Read the model definition and answer for the solid it produces. Units are mm, in the model's axes. A direction names the side the tool comes from. Coordinates: 2 decimals unless noted, no trailing zeros. Order: outer loops, then holes, each group sorted by start corner. A loop starts at its lowest first (then second) coordinate and runs counter-clockwise, first axis right, second up.
Autodesk Inventor part; units mm, degrees
ref_plane "YZ Plane" through (0, 0, 0) normal (1, 0, 0) x (0, 1, 0)
ref_plane "XZ Plane" through (0, 0, 0) normal (0, 1, 0) x (-1, 0, 0)
ref_plane "XY Plane" through (0, 0, 0) normal (0, 0, 1) x (1, 0, 0)
ref_plane "Work Plane1" through (0, 0, 0) normal (0, 0, 1) x (1, 0, 0)
sketch "Sketch1" plane through (0, 0, 0) normal (0, 0, 1) x (1, 0, 0)
  circle A0 centre (0, 24.15) radius 1.6 construction
  circle A1 centre (0, -24.15) radius 1.6 construction
  line L0 (-19.85, -7.6776) -> (-19.85, 7.6776) construction
  arc A2 (-19.85, -7.6776) -> (-19.2715, -9.0845) centre (-17.85, -7.6776) ccw construction
  line L1 (-2.2034, -26.3306) -> (-19.2715, -9.0845) construction
  arc A3 (-2.2034, -26.3306) -> (2.2034, -26.3306) centre (0, -24.15) ccw construction
  line L2 (19.2715, -9.0845) -> (2.2034, -26.3306) construction
  arc A4 (19.2715, -9.0845) -> (19.85, -7.6776) centre (17.85, -7.6776) ccw construction
  line L3 (19.85, 7.6776) -> (19.85, -7.6776) construction
  arc A5 (19.85, 7.6776) -> (19.2715, 9.0845) centre (17.85, 7.6776) ccw construction
  line L4 (2.2034, 26.3306) -> (19.2715, 9.0845) construction
  arc A6 (2.2034, 26.3306) -> (-2.2034, 26.3306) centre (0, 24.15) ccw construction
  line L5 (-19.2715, 9.0845) -> (-2.2034, 26.3306) construction
  arc A7 (-19.2715, 9.0845) -> (-19.85, 7.6776) centre (-17.85, 7.6776) ccw construction
  circle A8 centre (0, 0) radius 13.8 construction
  circle A9 centre (0, 0) radius 14.3 construction
  line L6 (-19.85, -27.25) -> (19.85, -27.25)
  line L7 (19.85, -27.25) -> (19.85, 27.25)
  line L8 (19.85, 27.25) -> (-19.85, 27.25)
  line L9 (-19.85, 27.25) -> (-19.85, -27.25)
  circle A10 centre (0, -24.15) radius 1.5
  circle A11 centre (0, 24.15) radius 1.5
  line L10 (14.85, 22.25) -> (14.85, -22.25)
  line L11 (14.85, -22.25) -> (-14.85, -22.25)
  line L12 (-14.85, -22.25) -> (-14.85, 22.25)
  line L13 (-14.85, 22.25) -> (14.85, 22.25)
  dimension "d0" = 0.5
  dimension "d2" = 3
  dimension "d3" = 3
  dimension "d4" = 5
extrude "Extrusion1" add sketch "Sketch1" along normal blind 50
sketch "Sketch2" plane through (-19.85, -27.25, 0) normal (-1, 0, 0) x (0, 0, 1)
  line L0 (50, 54.5) -> (50, 0)
  line L1 (50, 0) -> (50, 54.5)
  circle A0 centre (50, 27.25) radius 15
  point P0 (0, 27.25)
  point P1 (50, 12.25)
  point P2 (50, 42.25)
  dimension "d7" = 30
extrude "Extrusion2" cut sketch "Sketch2" against normal up to surface (34.7 mm away) contours L0 A0 picked at (45.0365, 27.8527)
sketch "Sketch3" plane through (0, 0, 50) normal (0, 0, 1) x (1, 0, 0)
  line L0 (19.85, 27.25) -> (-19.85, 27.25)
  line L1 (-19.85, 27.25) -> (19.85, 27.25)
  line L2 (19.85, 27.25) -> (19.85, 37.25)
  line L3 (19.85, 37.25) -> (-19.85, 37.25)
  line L4 (-19.85, 37.25) -> (-19.85, 27.25)
  line L5 (19.85, -27.25) -> (19.85, 27.25)
  circle A0 centre (-13.85, 32.25) radius 2.65
  circle A1 centre (13.85, 32.25) radius 2.65
  line L6 (0, 37.25) -> (0, 27.25) construction
  point P0 (0, 0)
  point P1 (-19.85, 32.25)
  dimension "d10" = 5.3
  dimension "d12" = 6
  dimension "d13" = 10
extrude "Extrusion3" add sketch "Sketch3" against normal blind 5
fillet "Fillet1" radius 2 1 edges at (0, 27.25, 45)
ref_plane "Work Plane2" through (-19.85, 0, 0) normal (0, 1, 0) x (1, 0, 0)
mirror "Mirror1" about plane through (-19.85, 0, 0) normal (0, 1, 0) of "Extrusion3", "Fillet1"
properties part number "peristaltic pump bracket"
1) Straight lines are drawn through the part: line 1 (Y direction, x = 0, z = 13); line 2 (Y direction, x = -13.85, z = 46.1); line 3 (Y direction, x = 2.5, z = 36). For each, find the intervals that lie inside material, in ascending order.
A:
line 1: y = -27.25 to -25.65, -22.65 to -22.25, 22.25 to 22.65, 25.65 to 27.25
line 2: y = -37.25 to -34.9, -29.6 to -22.25, 22.25 to 29.6, 34.9 to 37.25
line 3: y = -27.25 to -22.25, 22.25 to 27.25
2) A cutting plane is placed at C-C, the plane z = 33.5. Determine the outline of the cut face in (x, y).
A:
outline: (-19.85, -27.25) - (19.85, -27.25) - (19.85, 27.25) - (-19.85, 27.25) - close; hole (-14.85, -22.25) - (14.85, -22.25) - (14.85, 22.25) - (-14.85, 22.25) - close; hole circle Ø3 at (0, -24.15); hole circle Ø3 at (0, 24.15)
3) A cutting plane is placed at D-D, the plane y = -24.15. Determine the outline of the cut face in (x, z).
A:
outline: (-19.85, 0) - (-1.5, 0) - (-1.5, 50) - (-19.85, 50) - close; (1.5, 0) - (19.85, 0) - (19.85, 50) - (1.5, 50) - close
4) A cutting plane is placed at A-A, the plane x = 13.85. Determine the outline of the cut face in (y, z), and give its area (3 significant figures).
A:
outline: (-37.25, 45) - (-34.9, 45) - (-34.9, 50) - (-37.25, 50) - close; (-29.6, 45) - (-29.25, 45) arc R2 cw to (-27.25, 43) - (-27.25, 0) - (-22.25, 0) - (-22.25, 50) - (-29.6, 50) - close; (22.25, 0) - (27.25, 0) - (27.25, 43) arc R2 cw to (29.25, 45) - (29.6, 45) - (29.6, 50) - (22.25, 50) - close; (34.9, 45) - (37.25, 45) - (37.25, 50) - (34.9, 50) - close
area: 549 mm2
5) A cutting plane is placed at B-B, the plane y = 32.25. Determine the outline of the cut face in (x, z), and give its area (4 significant figures).
A:
outline: (-19.85, 45) - (-16.5, 45) - (-16.5, 50) - (-19.85, 50) - close; (-11.2, 45) - (11.2, 45) - (11.2, 50) - (-11.2, 50) - close; (16.5, 45) - (19.85, 45) - (19.85, 50) - (16.5, 50) - close
area: 145.5 mm2
6) Determine the mould class of faces 1 (the flat face through (0, 22.25, 25)), 2 (the flat face through (-19.85, 1, 25)), 3 (the flat face through (0, 27.25, 21)), 4 (the flat face through (19.85, -1, 25)) for opening direction X: pulls with the +X half, pulls with the -X half, needs draft (parallel to the pull), parting line crosses it, or undercut.
A:
face 1: undercut
face 2: pulls with the -X half
face 3: needs draft
face 4: pulls with the +X half
7) Which of the six approach directions +Z, -Z, +X, -X, +Y, -Y give full straight-line access (tool end or side, diameter ignored) to faces 5 (the flat face through (0, -27.25, 21)), 6 (the flat face through (0, 33, 45)), 7 (the flat face through (0, -22.25, 25))?
A:
face 5: -Z, +X, -X, -Y
face 6: -Z, +X, -X, +Y
face 7: +Z, -Z
8) Flat-ended cylindrical pins translate along their axes: pin 1 Ø8 at (x, y) = (-5, -16.5) entering from -Z; pin 2 Ø12 at (x, z) = (-2, 28) entering from -Y; pin 3 Ø6.5 at (x, y) = (-1, -34.5) entering from -Z; pin 4 Ø1 at (x, z) = (7.5, 19) entering from +Y. Find the tip coordinate at first contact, or state that the pin passes through.
A:
pin 1: passes through
pin 2: stops at y = -27.25
pin 3: stops at z = 45
pin 4: stops at y = 27.25
